```python
from build123d import *

# Parameters (mm, degrees)
SKETCH1_R           = 150
BOSS_EXTRUDE1_DEPTH = 100
CHAMFER1_SIZE       = 10
BOSS_EXTRUDE2_START = -100
BOSS_EXTRUDE2_DEPTH = 10
SKETCH3_R           = 5
CUT_EXTRUDE1_DEPTH  = 10
CIRPATTERN2_COUNT   = 3
SKETCH4_R           = 120
BOSS_EXTRUDE4_DEPTH = 15
BOSS_EXTRUDE4_TAPER = 30
SKETCH5_R           = 15
BOSS_EXTRUDE5_DEPTH = 30


with BuildPart() as part:
    # Sketch1 → Boss-Extrude1 (new body)
    with BuildSketch(Plane(origin=(0, 0, 0), x_dir=(1, 0, 0), z_dir=(0, 1, 0))):
        Circle(SKETCH1_R)
    extrude(amount=BOSS_EXTRUDE1_DEPTH)

    # Chamfer1
    chamfer1_edges = [part.edges().sort_by_distance(p)[0] for p in [
        (-150, 100, 0),
    ]]
    chamfer(chamfer1_edges, length=CHAMFER1_SIZE)

    # Sketch2 → Boss-Extrude2 (add)
    with BuildSketch(Plane(origin=(0, 100, 0), x_dir=(1, 0, 0), z_dir=(0, 1, 0)).offset(BOSS_EXTRUDE2_START)):
        with BuildLine():
            Line((-194.568322948, -40), (-194.568322948, 40))
            Line((-194.568322948, 40), (-144.568322948, 40))
            ThreePointArc((-144.568322948, 40), (-150, 0), (-144.568322948, -40))
            Line((-144.568322948, -40), (-194.568322948, -40))
        make_face()
    boss_extrude2 = extrude(amount=BOSS_EXTRUDE2_DEPTH)

    # Sketch3 → Cut-Extrude1 (cut)
    with BuildSketch(Plane(origin=(0, 10, 0), x_dir=(1, 0, 0), z_dir=(0, 1, 0))):
        with Locations((-172.284161474, -20)):
            Circle(SKETCH3_R)
        with Locations((-172.284161474, 20)):
            Circle(SKETCH3_R)
    cut_extrude1 = extrude(amount=-CUT_EXTRUDE1_DEPTH, mode=Mode.SUBTRACT)

    # CirPattern2: Boss-Extrude2, Cut-Extrude1 ×3 about axis
    cirpattern2_axis = Axis((0, 0, 0), (0, 1, 0))
    for i in range(1, CIRPATTERN2_COUNT):
        add(boss_extrude2.rotate(cirpattern2_axis, i * 360 / CIRPATTERN2_COUNT))
        add(cut_extrude1.rotate(cirpattern2_axis, i * 360 / CIRPATTERN2_COUNT), mode=Mode.SUBTRACT)

    # Sketch4 → Boss-Extrude4 (add)
    with BuildSketch(Plane(origin=(0, 100, 0), x_dir=(1, 0, 0), z_dir=(0, 1, 0))):
        Circle(SKETCH4_R)
    extrude(amount=BOSS_EXTRUDE4_DEPTH, taper=BOSS_EXTRUDE4_TAPER)

    # Sketch5 → Boss-Extrude5 (add)
    with BuildSketch(Plane(origin=(0, 115, 0), x_dir=(1, 0, 0), z_dir=(0, 1, 0))):
        Circle(SKETCH5_R)
    extrude(amount=BOSS_EXTRUDE5_DEPTH)


solid = part.part
```
Could you check a few things on this model? Use its own coordinates, in mm. A direction names the side the tool comes from. Coordinates: 2 decimals unless noted, no trailing zeros. Write each loop counter-clockwise with the first axis right and the second up, starting at its lowest first coordinate (ties: lowest second). Pieces come first, ordered by that corner, then holes. Notation, with made-up numbers: (-39, 87) -> (4, 87) arc R15 ccw to (4, 115) -> close; hole circle Ø9 at (-1, 22). An arc over 180 degrees is marked (long way). Return JSON: item names as keys, results as strings.
(1) I'm going to push flat-ended pins straight in: pin 1 (5 mm diameter, centred on x = -171, y = 6.5, fed in from +Z); pin 2 (5 mm diameter, centred on y = 59.5, z = -41, fed in from -X) (3 decimals); pin 3 (8 mm diameter, centred on x = -178.5, y = 2.5, fed in from -Z); pin 4 (9 mm diameter, centred on x = 68.82, z = 159.2, fed in from +Y). Where does each tip first touch, or does it pass through?
Numbers:
{"pin 1": "stops at z = 40", "pin 2": "stops at x = -144.975", "pin 3": "stops at z = -40", "pin 4": "passes through"}
(2) Imagine slicing it at A-A, the plane x = 0. Please give me the cut outline in (y, z), then the cut area to 3 significant figures.
Numbers:
{"outline": "(0, -150) -> (90, -150) -> (100, -140) -> (100, -120) -> (115, -111.34) -> (115, -15) -> (145, -15) -> (145, 15) -> (115, 15) -> (115, 111.34) -> (100, 120) -> (100, 140) -> (90, 150) -> (0, 150) -> close", "area": "34,300 mm2"}
(3) We'd pull the mould along Z, two halves only. Please class faces 1 (the flat face through (119.25, 4.93, 126.55)), 2 (the cylindrical face through (67.74, 5.07, -154.32)), 3 (the flat face through (49.97, 4.93, -166.55)), 4 (the cylindrical face through (-14.985, 129.79, -0.66)): +Z half, -Z half, draft (parallel to the pull), parting line (faces both ways), or undercut.
Numbers:
{"face 1": "undercut", "face 2": "undercut", "face 3": "-Z half", "face 4": "parting line"}
(4) Which directions (+Z, -Z, +X, -X, +Y, -Y) give clear straight access to the entire face, cutting with the end or side of a thin tool? Please do faces 5 (the cylindrical face through (-19.527, 44.37, -148.724)), 6 (the flat face through (85, 10, -146)), 7 (the flat face through (-169, 5, 40)), 8 (the flat face through (-194.568, 5, 1)).
Numbers:
{"face 5": "+Y", "face 6": "-Z, +X, +Y", "face 7": "+Z, -X, +Y, -Y", "face 8": "+Z, -Z, -X, +Y, -Y"}
(5) I need wall thicknesses on L1, parallel to Y at x = -37, z = 77; L2, parallel to X at y = 2.5, z = -20; L3, parallel to Y at x = 88.5, z = 161. Which ranges of each line are inside material? Lowest first, please.
Numbers:
{"L1": "y = 0 to 115", "L2": "x = -194.57 to -177.28, -167.28 to 148.66", "L3": "y = 0 to 10"}
(6) Imagine slicing it at B-B, the plane y = 31.5. Please give me the cut outline in (x, z), then the cut area to 3 significant figures.
Numbers:
{"outline": "circle Ø300 at (0, 0)", "area": "70,700 mm2"}
